```python
from build123d import *

# Parameters (mm, degrees)
SALIENTE_EXTRUIR1_DEPTH = 7.55
REDONDEO1_R             = 2
CROQUIS2_W              = 16.065204313
CROQUIS2_H              = 18
CORTAR_EXTRUIR1_DEPTH   = 2.5
CROQUIS3_R              = 5.5
CORTAR_EXTRUIR2_DEPTH   = 97.304594979
CROQUIS4_W              = 2
CROQUIS4_H              = 18
CORTAR_EXTRUIR3_DEPTH   = 6.5
CORTAR_EXTRUIR4_DEPTH   = 97.140912353


with BuildPart() as part:
    # Croquis1 → Saliente-Extruir1 (new body)
    with BuildSketch(Plane.XY):
        with BuildLine():
            Line((52.9, -7.25), (52.9, 64.75))
            ThreePointArc((52.9, 64.75), (58.9, 70.75), (64.9, 64.75))
            Line((64.9, 64.75), (64.9, -7.25))
            ThreePointArc((64.9, -7.25), (58.9, -13.25), (52.9, -7.25))
        make_face()
    extrude(amount=SALIENTE_EXTRUIR1_DEPTH)

    # Redondeo1
    redondeo1_edges = [part.edges().sort_by_distance(p)[0] for p in [
        (58.9, 70.75, 7.55),
        (64.9, 28.75, 7.55),
        (58.9, -13.25, 7.55),
        (52.9, 28.75, 7.55),
    ]]
    fillet(redondeo1_edges, radius=REDONDEO1_R)

    # Croquis2 → Cortar-Extruir1 (cut)
    with BuildSketch(Plane.XY.offset(7.55)):
        with Locations((54.867397844, 4.055228902)):
            Rectangle(CROQUIS2_W, CROQUIS2_H)
        with Locations((54.867397844, 53.444771098)):
            Rectangle(CROQUIS2_W, CROQUIS2_H)
    extrude(amount=-CORTAR_EXTRUIR1_DEPTH, mode=Mode.SUBTRACT)

    # Croquis3 → Cortar-Extruir2 (cut, through all)
    with BuildSketch(Plane.XY.offset(7.55)):
        with Locations((58.9, 28.75)):
            Circle(CROQUIS3_R)
    extrude(amount=-CORTAR_EXTRUIR2_DEPTH, mode=Mode.SUBTRACT)

    # Croquis4 → Cortar-Extruir3 (cut)
    with BuildSketch(Plane(origin=(64.9, 0, 0), x_dir=(0, 0, -1), z_dir=(1, 0, 0))):
        with Locations((-1.05, 4.055228902)):
            Rectangle(CROQUIS4_W, CROQUIS4_H)
        with Locations((-1.05, 53.444771098)):
            Rectangle(CROQUIS4_W, CROQUIS4_H)
    extrude(amount=-CORTAR_EXTRUIR3_DEPTH, mode=Mode.SUBTRACT)

    # Croquis5 → Cortar-Extruir4 (cut, through all)
    with BuildSketch(Plane.XY.offset(5.05)):
        with BuildLine():
            Line((62.541, 9.245228902), (62.541, -1.134771098))
            ThreePointArc((62.541, -1.134771098), (60.741, -2.934771098), (58.941, -1.134771098))
            Line((58.941, -1.134771098), (58.941, 9.245228902))
            ThreePointArc((58.941, 9.245228902), (60.741, 11.045228902), (62.541, 9.245228902))
        make_face()
        with BuildLine():
            Line((62.541, 48.254771098), (62.541, 58.634771098))
            ThreePointArc((62.541, 58.634771098), (60.741, 60.434771098), (58.941, 58.634771098))
            Line((58.941, 58.634771098), (58.941, 48.254771098))
            ThreePointArc((58.941, 48.254771098), (60.741, 46.454771098), (62.541, 48.254771098))
        make_face()
    extrude(amount=-CORTAR_EXTRUIR4_DEPTH, mode=Mode.SUBTRACT)


solid = part.part
```
CAD build for the part. Positions are in the model's coordinates, mm. A direction names the side the tool comes from. Give positions to 0.01 mm unless a question says otherwise; leave off trailing zeros. Order: outer loops, then holes, each group sorted by start corner. A loop starts at its lowest first (then second) coordinate and runs counter-clockwise, first axis right, second up.
(1) Flat gauge pins, fed straight in: pin 1 (2 mm diameter, centred on x = 61, z = 1.5, fed in from +Y); pin 2 (6 mm diameter, centred on x = 59, y = 57.5, fed in from +Z); pin 3 (2 mm diameter, centred on x = 61.5, z = 1.5, fed in from -Y). Where does each tip first touch, or does it go through?
(2) Drill centre lines: L1, parallel to X at y = 28.75, z = 3.25; L2, parallel to Y at x = 60.75, z = 1.25; L3, parallel to Y at x = 55.5, z = 5.5. Where is each one in solid material? Low to high.
(3) Saw through at A-A, the plane z = 3.5. Give the cut face in (x, y), then the cut area to 3 significant figures.
(4) Saw through at B-B, the plane y = 28.75. Give the cut face in (x, z).
(5) Mould opens along Y. For faces 6 (the flat face through (57, 4, 5.05)), 7 (the cylindrical face through (53.47, 63.61, 6.95)), 8 (the cylindrical face through (59.03, -13.25, 2.74)) say: released by +Y, released by -Y, zero draft, split by the parting line, or undercut.
(6) Tool access for faces 1 (the flat face through (59, 39, 7.55)), 2 (the flat face through (59, 20, 0)), 3 (the flat face through (63, 53, 2.05)), 4 (the flat face through (62.541, 4, 4)), 5 (the flat face through (62.9, 4, 6)): list every direction of +Z, -Z, +X, -X, +Y, -Y with a clear straight run to the whole face (end or side of a thin tool).
Results found:
1. pin 1: stops at y = 70.65
1. pin 2: stops at z = 5.05
1. pin 3: stops at y = -13.03
2. L1: x = 52.9 to 53.4, 64.4 to 64.9
2. L2: y = -12.96 to -4.94, 13.06 to 23.57, 33.93 to 44.44, 62.44 to 70.46
2. L3: y = -12.19 to -4.94, 13.06 to 24.43, 33.07 to 44.44, 62.44 to 69.69
3. outline: (52.9, -7.25) arc R6 ccw to (64.9, -7.25) - (64.9, 64.75) arc R6 ccw to (52.9, 64.75) - close; hole circle Ø11 at (58.9, 28.75); hole (58.94, -1.13) arc R1.8 ccw to (62.54, -1.13) - (62.54, 9.25) arc R1.8 ccw to (58.94, 9.25) - close; hole (58.94, 48.25) arc R1.8 ccw to (62.54, 48.25) - (62.54, 58.63) arc R1.8 ccw to (58.94, 58.63) - close
3. area: 787 mm2
4. outline: (52.9, 0) - (53.4, 0) - (53.4, 6.87) arc R2 ccw to (52.9, 5.55) - close; (64.4, 0) - (64.9, 0) - (64.9, 5.55) arc R2 ccw to (64.4, 6.87) - close
5. face 6: undercut
5. face 7: zero draft
5. face 8: released by -Y
6. face 1: +Z, +X, -X, +Y, -Y
6. face 2: -Z, +X, -X, +Y, -Y
6. face 3: +X
6. face 4: +Z, -Z
6. face 5: +Z, -X
